```python
from build123d import *

# Parameters (mm, degrees)
F0_W          = 17.715182
F0_H          = 7.343914
F1_DEPTH      = 25.4
F2_W          = 19.163959
F2_H          = 19.005526
F3_DEPTH      = 7.343914
F4_W          = 25.703696
F4_H          = 10.242827
F5_DEPTH      = 7.343914
F6_W          = 31.09887
F6_H          = 8.596847
F7_DEPTH      = 7.343914
F9_DEPTH      = 33.782
F9_DEPTH_BACK = 29.972


with BuildPart() as f1:
    # F0 (on Top) → F1 (new body)
    with BuildSketch(Plane.XY):
        with Locations((-19.371394, 23.481196)):
            Rectangle(F0_W, F0_H)
        Polygon((-45.126412, -19.809239), (-45.126412, 19.809239), (-28.228985, 19.809239), (-28.228985, 27.153153), (-54.209676, 27.153153), (-54.209676, -27.153153), (54.209676, -27.153153), (54.209676, 27.153153), (-10.513803, 27.153153), (-10.513803, 19.809239), (45.126412, 19.809239), (45.126412, -19.809239), align=None)
    extrude(amount=F1_DEPTH)

    # F2 (on face) → F3 (cut, through all)
    with BuildSketch(Plane.XZ.offset(27.153153)):
        with Locations((-23.425042, 9.502763)):
            Rectangle(F2_W, F2_H)
    extrude(amount=-F3_DEPTH, mode=Mode.SUBTRACT)

    # F4 (on face) → F5 (join, through all)
    with BuildSketch(Plane.XZ.offset(27.153153)):
        with Locations((27.443045, 12.561957)):
            Rectangle(F4_W, F4_H)
    extrude(amount=-F5_DEPTH)

    # F6 (on face) → F7 (cut, through all)
    with BuildSketch(Plane.XZ.offset(27.153153)):
        with Locations((26.846507, 12.30497)):
            Rectangle(F6_W, F6_H)
    extrude(amount=-F7_DEPTH, mode=Mode.SUBTRACT)

    # F8 (on Front) → F9 (join, two sides)
    with BuildSketch(Plane.XZ) as f9_sk:
        Polygon((-0.802159, 50.028846), (-58.465718, 25.240492), (59.17522, 25.240492), align=None)
    extrude(amount=F9_DEPTH)
    extrude(f9_sk.sketch, amount=-F9_DEPTH_BACK)


solid = f1.part
```
Input: part model. Units: mm. Frame: model coordinates. A direction names the side the tool comes from. Coordinates: 2 decimals unless noted, no trailing zeros. Write each loop counter-clockwise with the first axis right and the second up, starting at its lowest first coordinate (ties: lowest second). Pieces come first, ordered by that corner, then holes. Notation, with made-up numbers: (30.25, 87.25) -> (85.25, 87.25) arc R13 cw to (85.25, 95.25) -> close; hole circle Ø1 at (-39, 22.5). An arc over 180 degrees is marked (long way). Answer as a JSON object with one key per item and string values.
1. Section A-A on z = 24. Return the cut outline in (x, y).
Result set:
{"outline": "(-54.21, -27.15) -> (54.21, -27.15) -> (54.21, 27.15) -> (-54.21, 27.15) -> close; hole (-45.13, -19.81) -> (45.13, -19.81) -> (45.13, 19.81) -> (-45.13, 19.81) -> close"}
2. Mould query, pull axis X, two halves, no side actions, for faces 4 (the face through (-54.21, 0, 12)), 5 (the face through (0, -33.782, 35)), 6 (the face through (-1, 0, 25.24)). Classes: released by +X, released by -X, zero draft, split by the parting line, or undercut.
Result set:
{"face 4": "released by -X", "face 5": "zero draft", "face 6": "undercut"}
3. Access query for faces 1 (the face through (42.396, -24, 12)), 2 (the face through (-13.843, -24, 9)), 3 (the face through (-1, -27.153, 12)). Directions: +Z, -Z, +X, -X, +Y, -Y. A direction counts if a zero-diameter tool reaches every point of the face in a straight line with its end or side. Return the directions, or none.
Result set:
{"face 1": "-Y", "face 2": "-Z, -Y", "face 3": "-Z, +X, -X, -Y"}
4. Section D-D on z = 13. Return the cut outline in (x, y).
Result set:
{"outline": "(-54.21, -27.15) -> (-33.01, -27.15) -> (-33.01, -19.81) -> (-45.13, -19.81) -> (-45.13, 19.81) -> (45.13, 19.81) -> (45.13, -19.81) -> (42.4, -19.81) -> (42.4, -27.15) -> (54.21, -27.15) -> (54.21, 27.15) -> (-54.21, 27.15) -> close; (-13.84, -27.15) -> (11.3, -27.15) -> (11.3, -19.81) -> (-13.84, -19.81) -> close"}
5. Material intervals for line 1 (X direction, y = -6, z = 24.5); line 2 (Y direction, x = -40, z = 17); line 3 (X direction, y = 22, z = 4), sorted ascending. Write a range as from..to.
Result set:
{"line 1": "x = -54.21..-45.13, 45.13..54.21", "line 2": "y = -27.15..-19.81, 19.81..27.15", "line 3": "x = -54.21..54.21"}
6. First-contact query: P1, Ø12.5, axis at y = -2.5, z = 11.5, coming from the -X side; P2, Ø8, axis at x = 25.5, y = -22, coming from the +Z side; P3, Ø12, axis at y = -19, z = 40, coming from the -X side. Flat tips, straight axial feed; report the tip coordinate or a pass-through.
Result set:
{"P1": "stops at x = -54.21", "P2": "stops at z = 40.81", "P3": "stops at x = -38.09"}
7. Section C-C on x = 39.5. Return the cut outline in (y, z).
Result set:
{"outline": "(-33.78, 25.24) -> (-27.15, 25.24) -> (-27.15, 16.6) -> (-19.81, 16.6) -> (-19.81, 25.24) -> (19.81, 25.24) -> (19.81, 0) -> (27.15, 0) -> (27.15, 25.24) -> (29.97, 25.24) -> (29.97, 33.37) -> (-33.78, 33.37) -> close; (-27.15, 0) -> (-19.81, 0) -> (-19.81, 8.01) -> (-27.15, 8.01) -> close"}
8. Section B-B on y = 14.5. Return the cut outline in (x, z).
Result set:
{"outline": "(-58.47, 25.24) -> (-54.21, 25.24) -> (-54.21, 0) -> (-45.13, 0) -> (-45.13, 25.24) -> (45.13, 25.24) -> (45.13, 0) -> (54.21, 0) -> (54.21, 25.24) -> (59.18, 25.24) -> (-0.8, 50.03) -> close"}
